CAD build for the part. Positions are in the model's coordinates, mm. A direction names the side the tool comes from. Coordinates: 2 decimals unless noted, no trailing zeros. Order: outer loops, then holes, each group sorted by start corner. A loop starts at its lowest first (then second) coordinate and runs counter-clockwise, first axis right, second up. Notation, with made-up numbers: (85.25, -40) - (106.25, -40) arc R23 cw to (106.25, -14) - close; hole circle Ø8 at (-2.75, 20). An arc over 180 degrees is marked (long way). Write each question's results on one line, items separated by ' | '. Start each with the question number.
Q1. Pin check, flat tips, straight feed: P1, Ø2, axis at y = 26, z = 7.5, coming from the -X side; P2, Ø2, axis at x = 3, z = -29, coming from the +Y side; P3, Ø1.5, axis at y = 21, z = 2, coming from the +X side; P4, Ø8, axis at x = 22.5, y = 10.5, coming from the -Z side. Stop position of each tip, or through.
Q2. Pull direction Z, two halves, no side cores. Call faces 3 (the cylindrical face through (0.704, 31.992, -26.084)), 4 (the cylindrical face through (0.84, 37.99, 37.07)), 5 (the flat face through (-1, 28, -42)): released by +Z, released by -Z, zero draft, split by the parting line, or undercut.
Q3. Band-saw the part on A-A, the plane x = 0. Write the cut outline in (y, z), then the cut area to 3 significant figures.
Q4. Band-saw the part on D-D, the plane y = 21. Write the cut outline in (x, z).
Q5. Wall check: probe 1 along Z at (x, y) = (0, 28); probe 2 along Z at (x, y) = (27, 21); probe 3 along X at (y, z) = (27.5, 0). Give the ranges that are in metal, low to high.
Q6. Band-saw the part on B-B, the plane z = 0. Write the cut outline in (x, y), then the cut area to 3 significant figures.
Q7. Band-saw the part on C-C, the plane y = 28. Write the cut outline in (x, z).
Q8. Which spindle directions (+Z, -Z, +X, -X, +Y, -Y) get a long thin tool onto all of the face, cutting with end or side? Do faces 1 (the cylindrical face through (3, 27, 0)), 2 (the cylindrical face through (0.66, 29.993, 4.724)). Say none if no direction does.
```python
from build123d import *

# Parameters (mm, degrees)
REVOLVE1_START     = -42
REVOLVE1_DEPTH     = 42
REVOLVE1_2_DEPTH   = 10
REVOLVE1_START_2   = -32
REVOLVE1_3_DEPTH   = 12
SKETCH3_R          = 3
CUT_EXTRUDE1_DEPTH = 65.093681436


# Read off the part's stored shape, not the designer's step: Revolve1
with BuildPart() as part:
    # Revolve1 outline → Revolve1 (new body)
    with BuildSketch(Plane.XY.offset(REVOLVE1_START)):
        with BuildLine():
            ThreePointArc((-25, 0), (0, 25), (25, 0))
            Line((25, 0), (30, 0))
            ThreePointArc((30, 0), (0, 30), (-30, 0))
            Line((-30, 0), (-25, 0))
        make_face()
    revolve1 = extrude(amount=REVOLVE1_DEPTH)



with BuildPart() as body_2:
    # Revolve1 2 outline → Revolve1 2 (new body)
    with BuildSketch(Plane.XY.offset(REVOLVE1_START)):
        with BuildLine():
            ThreePointArc((-30, 0), (0, 30), (30, 0))
            Line((30, 0), (38, 0))
            ThreePointArc((38, 0), (0, 38), (-38, 0))
            Line((-38, 0), (-30, 0))
        make_face()
    revolve1_2 = extrude(amount=REVOLVE1_2_DEPTH)


with BuildPart() as part_1:
    add(part.part)

    add(body_2.part)  # Revolve1 3 merges body 2
    # Revolve1 3 outline → Revolve1 3 (add)
    with BuildSketch(Plane.XY.offset(REVOLVE1_START_2)):
        with BuildLine():
            ThreePointArc((-30, 0), (0, 30), (30, 0))
            Line((30, 0), (32, 0))
            ThreePointArc((32, 0), (0, 32), (-32, 0))
            Line((-32, 0), (-30, 0))
        make_face()
    revolve1_3 = extrude(amount=REVOLVE1_3_DEPTH)

    # Mirror1: Revolve1, Revolve1 2, Revolve1 3 across plane
    add(revolve1.mirror(Plane(origin=(30, 0, 0), x_dir=(1, 0, 0), z_dir=(0, 0, -1))))
    add(revolve1_2.mirror(Plane(origin=(30, 0, 0), x_dir=(1, 0, 0), z_dir=(0, 0, -1))))
    add(revolve1_3.mirror(Plane(origin=(30, 0, 0), x_dir=(1, 0, 0), z_dir=(0, 0, -1))))

    # Sketch3 → Cut-Extrude1 (cut, through all)
    with BuildSketch(Plane(origin=(0, 30, 0), x_dir=(1, 0, 0), z_dir=(0, 1, 0))):
        with Locations(Location((0, 0, 0), (0, 0, 270))):
            Circle(SKETCH3_R)
    extrude(amount=-CUT_EXTRUDE1_DEPTH, mode=Mode.SUBTRACT)


solid = part_1.part
```
Results below:
1) P1: stops at x = -16.58 | P2: stops at y = 31.94 | P3: stops at x = 22.13 | P4: stops at z = -42
2) face 3: undercut | face 4: zero draft | face 5: released by -Z
3) outline: (25, -42) - (38, -42) - (38, -32) - (32, -32) - (32, -20) - (30, -20) - (30, -3) - (25, -3) - close; (25, 3) - (30, 3) - (30, 20) - (32, 20) - (32, 32) - (38, 32) - (38, 42) - (25, 42) - close | area: 598 mm²
4) outline: (-31.67, -42) - (-13.56, -42) - (-13.56, 42) - (-31.67, 42) - (-31.67, 32) - (-24.15, 32) - (-24.15, 20) - (-21.42, 20) - (-21.42, -20) - (-24.15, -20) - (-24.15, -32) - (-31.67, -32) - close; (13.56, -42) - (31.67, -42) - (31.67, -32) - (24.15, -32) - (24.15, -20) - (21.42, -20) - (21.42, 20) - (24.15, 20) - (24.15, 32) - (31.67, 32) - (31.67, 42) - (13.56, 42) - close
5) probe 1: z = -42 to -3, 3 to 42 | probe 2: z = -42 to -32, 32 to 42 | probe 3: x = -11.99 to -3, 3 to 11.99
6) outline: (-30, 0) - (-25, 0) arc R25 cw to (-3, 24.82) - (-3, 29.85) arc R30 ccw to start; (3, 24.82) arc R25 cw to (25, 0) - (30, 0) arc R30 ccw to (3, 29.85) - close | area: 402 mm²
7) outline: (-25.69, -42) - (25.69, -42) - (25.69, -32) - (15.49, -32) - (15.49, -20) - (10.77, -20) - (10.77, 20) - (15.49, 20) - (15.49, 32) - (25.69, 32) - (25.69, 42) - (-25.69, 42) - (-25.69, 32) - (-15.49, 32) - (-15.49, 20) - (-10.77, 20) - (-10.77, -20) - (-15.49, -20) - (-15.49, -32) - (-25.69, -32) - close; hole circle Ø6 at (0, 0)
8) face 1: +Y, -Y | face 2: +Y
